Can you work these out from the model? Positions are in its coordinate system, mm. Face numbers are marked on the shaded views. A direction names the side the tool comes from. Coordinates: 2 decimals unless noted, no trailing zeros. Order: outer loops, then holes, each group sorted by start corner. A loop starts at its lowest first (then second) coordinate and runs counter-clockwise, first axis right, second up. Notation, with made-up numbers: (44, -36) -> (69, -36) arc R15 cw to (69, -22) -> close; hole circle Ø8 at (-1, 76). An arc over 180 degrees is marked (long way). Answer in a Markdown table with one row per item. Add a question column.
1. On a 3-axis mill with a long thin cutter (end or side, diameter ignored), from which of +Z, -Z, +X, -X, +Y, -Y can I reach the whole of each face in a straight line? I mean the marked faces 1, 2, 3 and 4. Say none if no direction works.
2. If I drill on line 1 along Z through (x, y) = (9, 7.5); line 2 along Y through (x, z) = (-6.5, 1.75); line 3 along Z through (x, y) = (9.5, 0), over which ranges is the centre line in solid material (lowest first)? Write a range as [from, to].
3. Imagine slicing it at A-A on y = 0. Write out the boundary of the cut face in (x, z).
4. We'd pull the mould along Y, two halves only. Please class the marked faces 5, 6, 7 and 8: pulls with the +Y half, pulls with the -Y half, needs draft (parallel to the pull), parting line crosses it, or undercut.
5. Imagine slicing it at D-D on x = -10. Write out the boundary of the cut face in (y, z).
6. Imagine slicing it at C-C on z = 7.75. Write out the boundary of the cut face in (x, y), plus the area to 3 significant figures.
7. Imagine slicing it at B-B on x = 0. Write out the boundary of the cut face in (y, z), plus the area to 3 significant figures.
8. Will these pins go through, and if not, where does the flat tip stop? pin 1 (4.5 mm diameter, centred on y = -0.5, z = 6.5, fed in from -X); pin 2 (9.5 mm diameter, centred on x = 2, y = 1, fed in from +Z); pin 3 (7 mm diameter, centred on x = -9, z = 11.5, fed in from +Y).
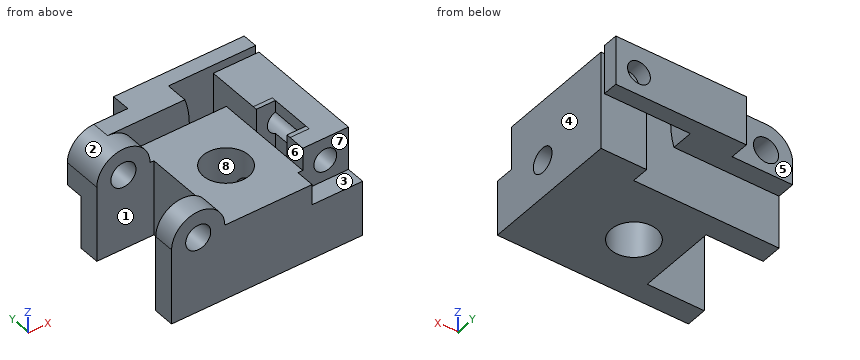
from build123d import *

# Parameters (mm, degrees)
SZKIC2_W                     = 17.619731325
SZKIC2_H                     = 16
SZKIC2_R                     = 3
DODANIE_WYCI_GNI_CIE1_DEPTH  = 10
SZKIC3_R                     = 1.65
WYTNIJ_WYCI_GNI_CIE1_DEPTH   = 10
WYTNIJ_WYCI_GNI_CIE2_DEPTH   = 2.5
DODANIE_WYCI_GNI_CIE2_DEPTH  = 2.5
SZKIC7_R                     = 1.65
DODANIE_WYCI_GNI_CIE4_DEPTH  = 2.8
SZKIC10_R                    = 1.65
DODANIE_WYCI_GNI_CIE5_DEPTH  = 2.9
SZKIC11_R                    = 1.65
DODANIE_WYCI_GNI_CIE6_DEPTH  = 2
SZKIC12_W                    = 6
SZKIC12_H                    = 13
DODANIE_WYCI_GNI_CIE7_DEPTH  = 2.3
SZKIC16_W                    = 6
SZKIC16_H                    = 3
DODANIE_WYCI_GNI_CIE12_DEPTH = 4.75
SZKIC17_W                    = 3.5
SZKIC17_H                    = 3
DODANIE_WYCI_GNI_CIE13_DEPTH = 6.5
SZKIC18_W                    = 6
SZKIC18_H                    = 3.354251662
DODANIE_WYCI_GNI_CIE14_DEPTH = 4.75
WYTNIJ_WYCI_GNI_CIE3_REACH   = 30.128
SZKIC19_R                    = 1.181229449
SZKIC21_W                    = 2.5
SZKIC21_H                    = 0.556642191
DODANIE_WYCI_GNI_CIE15_DEPTH = 11.418457
WYTNIJ_WYCI_GNI_CIE4_START   = -18.3
SZKIC22_R                    = 1.181229449
WYTNIJ_WYCI_GNI_CIE4_DEPTH   = 18.3
SZKIC34_W                    = 7.949380073
SZKIC34_H                    = 6.5
WYTNIJ_WYCI_GNI_CIE5_DEPTH   = 2.5
SZKIC35_W                    = 6.6400164
SZKIC35_H                    = 5.717036495
WYTNIJ_WYCI_GNI_CIE6_DEPTH   = 2.5
SZKIC36_R                    = 1.5
WYTNIJ_WYCI_GNI_CIE7_DEPTH   = 21


with BuildPart() as part:
    # Szkic2 → Dodanie-wyciągnięcie1 (new body)
    with BuildSketch(Plane.XY):
        with Locations((3.190134337, 0)):
            Rectangle(SZKIC2_W, SZKIC2_H)
        Circle(SZKIC2_R, mode=Mode.SUBTRACT)
    extrude(amount=DODANIE_WYCI_GNI_CIE1_DEPTH)

    # Szkic3 → Wytnij-wyciągnięcie1 (cut)
    with BuildSketch(Plane(origin=(12, 0, 0), x_dir=(0, 0, -1), z_dir=(1, 0, 0))):
        with Locations(Location((-5, 0, 0), (0, 0, 90))):
            Circle(SZKIC3_R)
    extrude(amount=-WYTNIJ_WYCI_GNI_CIE1_DEPTH, mode=Mode.SUBTRACT)

    # Szkic5 → Wytnij-wyciągnięcie2 (cut)
    with BuildSketch(Plane(origin=(6, 0, 0), x_dir=(0, 0, -1), z_dir=(1, 0, 0))):
        Polygon((-8.418457275, 3.25), (-10, 3.25), (-10, -3.25), (-8.418457275, -3.25), (-1.581542725, -3.25), (-1.581542725, 3.25), align=None)
    extrude(amount=WYTNIJ_WYCI_GNI_CIE2_DEPTH, mode=Mode.SUBTRACT)

    # Szkic6 → Dodanie-wyciągnięcie2 (add)
    with BuildSketch(Plane(origin=(6, 0, 0), x_dir=(0, 0, -1), z_dir=(1, 0, 0))):
        Polygon((-1.591079408, 3.256272654), (-1.591079408, 0.295576336), (-3.210214166, 3.1), (-3.210214166, 3.256272654), align=None)
    dodanie_wyci_gni_cie2 = extrude(amount=DODANIE_WYCI_GNI_CIE2_DEPTH)

    # Lustro1: Dodanie-wyciągnięcie2 across plane
    add(dodanie_wyci_gni_cie2.mirror(Plane.ZX))

    # Szkic7 → Dodanie-wyciągnięcie4 (add)
    with BuildSketch(Plane.XZ.offset(8)):
        with BuildLine():
            Line((-13.119731325, 10), (-13.119731325, 0))
            Line((-13.119731325, 0), (-5.619731325, 0))
            Line((-5.619731325, 0), (-5.619731325, 10))
            Line((-5.619731325, 10), (-6.119731325, 10))
            ThreePointArc((-6.119731325, 10), (-9.619731325, 13.5), (-13.119731325, 10))
        make_face()
        with Locations(Location((-9.619731325, 10, 0), (0, 0, 270))):
            Circle(SZKIC7_R, mode=Mode.SUBTRACT)
    dodanie_wyci_gni_cie4 = extrude(amount=-DODANIE_WYCI_GNI_CIE4_DEPTH)

    # Lustro2: Dodanie-wyciągnięcie4 across plane
    add(dodanie_wyci_gni_cie4.mirror(Plane.ZX))

    # Szkic10 → Dodanie-wyciągnięcie5 (add)
    with BuildSketch(Plane(origin=(0, 8, 0), x_dir=(1, 0, 0), z_dir=(0, 1, 0))):
        with BuildLine():
            Line((-6.119731325, -13.5), (0.54454435, -13.5))
            ThreePointArc((0.54454435, -13.5), (1.127068602, -10.262281002), (0.703180086, -7))
            Line((0.703180086, -7), (-6.119731325, -7))
            Line((-6.119731325, -7), (-13.119731325, -7))
            Line((-13.119731325, -7), (-13.119731325, -10))
            ThreePointArc((-13.119731325, -10), (-12.094605059, -12.474873734), (-9.619731325, -13.5))
            Line((-9.619731325, -13.5), (-6.119731325, -13.5))
        make_face()
        with Locations(Location((-9.619731325, -10, 0), (0, 0, 90))):
            Circle(SZKIC10_R, mode=Mode.SUBTRACT)
    extrude(amount=DODANIE_WYCI_GNI_CIE5_DEPTH)

    # Szkic11 → Dodanie-wyciągnięcie6 (add)
    with BuildSketch(Plane(origin=(0, 10.9, 0), x_dir=(1, 0, 0), z_dir=(0, 1, 0))):
        with BuildLine():
            Line((12, -7), (-13.119731325, -7))
            Line((-13.119731325, -7), (-13.119731325, -10))
            ThreePointArc((-13.119731325, -10), (-12.094605059, -12.474873734), (-9.619731325, -13.5))
            Line((-9.619731325, -13.5), (12, -13.5))
            Line((12, -13.5), (12, -7))
        make_face()
        with Locations(Location((-9.619731325, -10, 0), (0, 0, 90))):
            Circle(SZKIC11_R, mode=Mode.SUBTRACT)
    extrude(amount=DODANIE_WYCI_GNI_CIE6_DEPTH)

    # Szkic12 → Dodanie-wyciągnięcie7 (add)
    with BuildSketch(Plane(origin=(0, 8, 0), x_dir=(1, 0, 0), z_dir=(0, 1, 0))):
        with Locations((9, -6.5)):
            Rectangle(SZKIC12_W, SZKIC12_H)
    extrude(amount=DODANIE_WYCI_GNI_CIE7_DEPTH)

    # Szkic16 → Dodanie-wyciągnięcie12 (add)
    with BuildSketch(Plane.XZ.offset(-8)):
        with Locations((9, 11.5)):
            Rectangle(SZKIC16_W, SZKIC16_H)
    extrude(amount=DODANIE_WYCI_GNI_CIE12_DEPTH)

    # Szkic17 → Dodanie-wyciągnięcie13 (add)
    with BuildSketch(Plane.XZ.offset(-3.25)):
        with Locations((10.25, 11.5)):
            Rectangle(SZKIC17_W, SZKIC17_H)
    extrude(amount=DODANIE_WYCI_GNI_CIE13_DEPTH)

    # Szkic18 → Dodanie-wyciągnięcie14 (add)
    with BuildSketch(Plane.XZ.offset(3.25)):
        with Locations((9, 11.322874169)):
            Rectangle(SZKIC18_W, SZKIC18_H)
    extrude(amount=DODANIE_WYCI_GNI_CIE14_DEPTH)

    # Wytnij-wyciągnięcie3: up to this face of the body (flat: up to its plane)
    wytnij_wyci_gni_cie3_end = Plane(part.part.faces().sort_by_distance((-0.291063064, -8, 5.711108324))[0])
    # Szkic19 → Wytnij-wyciągnięcie3 (cut, up to the picked face)
    with BuildSketch(Plane(origin=(0, 12.9, 0), x_dir=(1, 0, 0), z_dir=(0, 1, 0)), mode=Mode.PRIVATE) as wytnij_wyci_gni_cie3_sk1:
        with Locations(Location((9, -10, 0), (0, 0, 270))):
            Circle(SZKIC19_R)
    wytnij_wyci_gni_cie3_tool1 = split(extrude(wytnij_wyci_gni_cie3_sk1.sketch, amount=-WYTNIJ_WYCI_GNI_CIE3_REACH, mode=Mode.PRIVATE), bisect_by=wytnij_wyci_gni_cie3_end, keep=Keep.BOTH, mode=Mode.PRIVATE)
    add(wytnij_wyci_gni_cie3_tool1.solids().sort_by(Axis((9, 12.9, 10), (0, -1, 0)))[0], mode=Mode.SUBTRACT)

    # Szkic21 → Dodanie-wyciągnięcie15 (add)
    with BuildSketch(Plane.XY.offset(1.581542725)):
        with Locations((7.25, 2.978321096)):
            Rectangle(SZKIC21_W, SZKIC21_H)
    dodanie_wyci_gni_cie15 = extrude(amount=DODANIE_WYCI_GNI_CIE15_DEPTH)

    # Lustro3: Dodanie-wyciągnięcie15 across plane
    add(dodanie_wyci_gni_cie15.mirror(Plane.ZX))

    # Szkic22 → Wytnij-wyciągnięcie4 (cut)
    with BuildSketch(Plane.XZ.offset(8).offset(WYTNIJ_WYCI_GNI_CIE4_START)):
        with Locations(Location((9, 10, 0), (0, 0, 90))):
            Circle(SZKIC22_R)
    extrude(amount=WYTNIJ_WYCI_GNI_CIE4_DEPTH, mode=Mode.SUBTRACT)

    # Szkic34 → Wytnij-wyciągnięcie5 (cut)
    with BuildSketch(Plane(origin=(0, 12.9, 0), x_dir=(1, 0, 0), z_dir=(0, 1, 0))):
        with Locations((-9.145041288, -10.25)):
            Rectangle(SZKIC34_W, SZKIC34_H)
    extrude(amount=-WYTNIJ_WYCI_GNI_CIE5_DEPTH, mode=Mode.SUBTRACT)

    # Szkic35 → Wytnij-wyciągnięcie6 (cut)
    with BuildSketch(Plane.XZ.offset(8)):
        with Locations((8.6799918, 10.141481753)):
            Rectangle(SZKIC35_W, SZKIC35_H)
    extrude(amount=-WYTNIJ_WYCI_GNI_CIE6_DEPTH, mode=Mode.SUBTRACT)

    # Szkic36 → Wytnij-wyciągnięcie7 (cut)
    with BuildSketch(Plane(origin=(0, 15, 0), x_dir=(1, 0, 0), z_dir=(0, 1, 0))):
        with Locations(Location((8.94965168, -10.000267868, 0), (0, 0, 270))):
            Circle(SZKIC36_R)
    extrude(amount=-WYTNIJ_WYCI_GNI_CIE7_DEPTH, mode=Mode.SUBTRACT)


solid = part.part
Answers follow:
| question | item | result |
|---|---|---|
| 1 | face 1 | +Z, -Z, -X |
| 1 | face 2 | +Z, -Y |
| 1 | face 3 | +Z, +X, -Y |
| 1 | face 4 | +Z, -Z, +X, +Y, -Y |
| 2 | line 1 | z = [0, 8.5], [11.5, 13] |
| 2 | line 2 | y = [-8, -5.2], [5.2, 8] |
| 2 | line 3 | z = [0, 3.35], [6.65, 8.6], [11.4, 13] |
| 3 | outline | (-5.62, 0) -> (-3, 0) -> (-3, 10) -> (-5.62, 10) -> close; (3, 0) -> (12, 0) -> (12, 3.35) -> (8.5, 3.35) -> (8.5, 1.58) -> (6, 1.58) -> (6, 3.35) -> (3, 3.35) -> close; (3, 6.65) -> (6, 6.65) -> (6, 10) -> (3, 10) -> close; (8.5, 6.65) -> (12, 6.65) -> (12, 13) -> (8.5, 13) -> (8.5, 11.43) arc R1.5 cw (long way) to (8.5, 8.57) -> close |
| 4 | face 5 | pulls with the +Y half |
| 4 | face 6 | needs draft |
| 4 | face 7 | pulls with the -Y half |
| 4 | face 8 | undercut |
| 5 | outline | (-8, 0) -> (-5.2, 0) -> (-5.2, 8.39) -> (-8, 8.39) -> close; (-8, 11.61) -> (-5.2, 11.61) -> (-5.2, 13.48) -> (-8, 13.48) -> close; (5.2, 0) -> (8, 0) -> (8, 7) -> (10.4, 7) -> (10.4, 8.39) -> (5.2, 8.39) -> close; (5.2, 11.61) -> (10.4, 11.61) -> (10.4, 13.48) -> (5.2, 13.48) -> close |
| 6 | outline | (-13.12, -8) -> (5.36, -8) -> (5.36, -5.5) -> (12, -5.5) -> (12, 10.3) -> (6, 10.3) -> (6, 8) -> (0.89, 8) -> (0.89, 10.9) -> (12, 10.9) -> (12, 12.9) -> (-5.17, 12.9) -> (-5.17, 10.4) -> (-13.12, 10.4) -> (-13.12, 5.2) -> (-5.62, 5.2) -> (-5.62, -5.2) -> (-13.12, -5.2) -> close; hole circle Ø6 at (0, 0); hole (6, -2.7) -> (8.5, -2.7) -> (8.5, 2.7) -> (6, 2.7) -> close |
| 6 | area | 350 mm² |
| 7 | outline | (-8, 0) -> (-3, 0) -> (-3, 10) -> (-8, 10) -> close; (3, 0) -> (8, 0) -> (8, 7) -> (12.9, 7) -> (12.9, 13.5) -> (8, 13.5) -> (8, 10) -> (3, 10) -> close |
| 7 | area | 132 mm² |
| 8 | pin 1 | stops at x = -5.62 |
| 8 | pin 2 | stops at z = 13 |
| 8 | pin 3 | stops at y = 10.4 |
